from build123d import *

# Parameters (mm, degrees)
BASE_FLANGE1_DEPTH = 40
SKETCH2_R          = 1.5
SKETCH2_W          = 12.8
SKETCH2_H          = 3.5
SKETCH2_H_2        = 2
SKETCH2_H_3        = 4
SKETCH2_W_2        = 2
SKETCH2_H_4        = 9.5
CUT_EXTRUDE1_DEPTH = 33.4
CUT_EXTRUDE2_REACH = 68.173
SKETCH4_R          = 2


# Sheet-metal steps are written as plain solids
with BuildPart() as part:
    # Sketch1 → Base-Flange1 (new body)
    with BuildSketch(Plane(origin=(0, 0, 0), x_dir=(1, 0, 0), z_dir=(0, 1, 0))):
        with BuildLine():
            Line((14.7, 24), (14.7, -23.2634))
            ThreePointArc((14.7, -23.2634), (14.484254855, -23.784254855), (13.9634, -24))
            Line((13.9634, -24), (-13.9634, -24))
            ThreePointArc((-13.9634, -24), (-14.484254855, -23.784254855), (-14.7, -23.2634))
            Line((-14.7, -23.2634), (-14.7, 24))
            Line((-14.7, 24), (-16.7, 24))
            Line((-16.7, 24), (-16.7, -23.2634))
            ThreePointArc((-16.7, -23.2634), (-15.898468417, -25.198468417), (-13.9634, -26))
            Line((-13.9634, -26), (13.9634, -26))
            ThreePointArc((13.9634, -26), (15.898468417, -25.198468417), (16.7, -23.2634))
            Line((16.7, -23.2634), (16.7, 24))
            Line((16.7, 24), (14.7, 24))
        make_face()
    extrude(amount=BASE_FLANGE1_DEPTH)

    # Sketch2 → Cut-Extrude1 (cut)
    with BuildSketch(Plane.ZY.offset(16.7)):
        with Locations((-16.25, 12)):
            Circle(SKETCH2_R)
        with Locations((-16.25, 28)):
            Circle(SKETCH2_R)
        with Locations((21, 4)):
            Circle(SKETCH2_R)
        with Locations((21, 36)):
            Circle(SKETCH2_R)
        with Locations((-11, 4)):
            Circle(SKETCH2_R)
        with Locations((-11, 36)):
            Circle(SKETCH2_R)
        with Locations((10.15, 36)):
            Rectangle(SKETCH2_W, SKETCH2_H)
        with Locations((10.15, 17.5)):
            Rectangle(SKETCH2_W, SKETCH2_H_2)
        with Locations((10.15, 11)):
            Rectangle(SKETCH2_W, SKETCH2_H_3)
        with Locations((10.15, 29)):
            Rectangle(SKETCH2_W, SKETCH2_H_3)
        with Locations((10.15, 4)):
            Rectangle(SKETCH2_W, SKETCH2_H)
        with Locations((10.15, 22.5)):
            Rectangle(SKETCH2_W, SKETCH2_H_2)
        with Locations((-19.25, 8.75)):
            Rectangle(SKETCH2_W_2, SKETCH2_H_4)
        with Locations((-19.25, 31.25)):
            Rectangle(SKETCH2_W_2, SKETCH2_H_4)
    extrude(amount=-CUT_EXTRUDE1_DEPTH, mode=Mode.SUBTRACT)

    # Sketch4 → Cut-Extrude2 (cut, up to next)
    with BuildSketch(Plane.XY.offset(26), mode=Mode.PRIVATE) as cut_extrude2_sk1:
        with Locations((0, 10)):
            Circle(SKETCH4_R)
    cut_extrude2_tool1 = extrude(cut_extrude2_sk1.sketch, amount=-CUT_EXTRUDE2_REACH, mode=Mode.PRIVATE) & part.part
    # Sketch4 → Cut-Extrude2 (cut, up to next)
    with BuildSketch(Plane.XY.offset(26), mode=Mode.PRIVATE) as cut_extrude2_sk2:
        with Locations((0, 30)):
            Circle(SKETCH4_R)
    cut_extrude2_tool2 = extrude(cut_extrude2_sk2.sketch, amount=-CUT_EXTRUDE2_REACH, mode=Mode.PRIVATE) & part.part
    add(cut_extrude2_tool1.solids().sort_by_distance((0, 10, 26))[0], mode=Mode.SUBTRACT)
    add(cut_extrude2_tool2.solids().sort_by_distance((0, 30, 26))[0], mode=Mode.SUBTRACT)


solid = part.part
Verification items for the finished model (mm, model axes). A direction names the side the tool comes from. Round coordinates to 2 decimals unless told otherwise and drop trailing zeros. Loops run counter-clockwise (first coordinate to the right, second up) from the corner with the lowest first, then second, coordinate; pieces in that order, holes last. Notation, with made-up numbers: (88.5, 83.5) - (94.5, 83.5) arc R31 ccw to (94.5, 118.5) - close; hole circle Ø2 at (23.5, 75). An arc over 180 degrees is marked (long way). Answer in a Markdown table with one row per item. Add a question column.
Q1. Section check B-B on x = 0. Enter the section's corners in (y, z), plus the area to 3 significant figures.
Q2. Section check A-A on z = -11. Enter the section's corners in (x, y).
Q3. Tool access check on faces 1 (the face through (16, 20, -24)), 2 (the face through (-16, 31, 10)), 3 (the face through (14.7, 20, -1)). Record the directions out of +Z, -Z, +X, -X, +Y, -Y that give a thin tool (end or side, any length) a straight path to the whole face; none if there is none.
Q4. Section check C-C on z = 8.5. State how many separate pieces and enclosed holes the cut face has, plus the area to 3 significant figures.
Q5. Gauge pin test, flat ends, axial feed: pin 1 (1 mm diameter, centred on x = -1.5, y = 21, fed in from -Z); pin 2 (8 mm diameter, centred on x = -10.5, y = 27, fed in from -Z); pin 3 (1.6 mm diameter, centred on x = -15.5, y = 36.5, fed in from +Z). Record the tip position at first contact, or that the pin passes through.
Q6. Section check D-D on z = -16.5. Enter the section's corners in (x, y), plus the area to 3 significant figures.
Q7. Release check for a two-part mould opening along Z. For faces 4 (the face through (-15, 40, 5)), 5 (the face through (16, 27, 10)), 6 (the face through (-15.92, 19.72, 25.177)) record: pulls with the +Z half, pulls with the -Z half, needs draft (parallel to the pull), parting line crosses it, or undercut.
Q8. Material ranges on line 1 (Y direction, x = 15.4, z = -11); line 2 (X direction, y = 33, z = 10.5); line 3 (Y direction, x = 16, z = -16), recorded low to high.
Found:
| question | item | result |
|---|---|---|
| 1 | outline | (0, 24) - (8, 24) - (8, 26) - (0, 26) - close; (12, 24) - (28, 24) - (28, 26) - (12, 26) - close; (32, 24) - (40, 24) - (40, 26) - (32, 26) - close |
| 1 | area | 64.0 mm² |
| 2 | outline | (-16.7, 0) - (-14.7, 0) - (-14.7, 2.5) - (-16.7, 2.5) - close; (-16.7, 5.5) - (-14.7, 5.5) - (-14.7, 34.5) - (-16.7, 34.5) - close; (-16.7, 37.5) - (-14.7, 37.5) - (-14.7, 40) - (-16.7, 40) - close; (14.7, 0) - (16.7, 0) - (16.7, 2.5) - (14.7, 2.5) - close; (14.7, 5.5) - (16.7, 5.5) - (16.7, 34.5) - (14.7, 34.5) - close; (14.7, 37.5) - (16.7, 37.5) - (16.7, 40) - (14.7, 40) - close |
| 3 | face 1 | -Z, +X, -X, +Y, -Y |
| 3 | face 2 | +X, -X |
| 3 | face 3 | -Z, +Y, -Y |
| 4 | separate pieces | 14 |
| 4 | enclosed holes | 0 |
| 4 | area | 84.0 mm² |
| 5 | pin 1 | stops at z = 24 |
| 5 | pin 2 | stops at z = 23.77 |
| 5 | pin 3 | stops at z = 25.9 |
| 6 | outline | (-16.7, 0) - (-14.7, 0) - (-14.7, 10.52) - (-16.7, 10.52) - close; (-16.7, 13.48) - (-14.7, 13.48) - (-14.7, 26.52) - (-16.7, 26.52) - close; (-16.7, 29.48) - (-14.7, 29.48) - (-14.7, 40) - (-16.7, 40) - close; (14.7, 0) - (16.7, 0) - (16.7, 10.52) - (14.7, 10.52) - close; (14.7, 13.48) - (16.7, 13.48) - (16.7, 26.52) - (14.7, 26.52) - close; (14.7, 29.48) - (16.7, 29.48) - (16.7, 40) - (14.7, 40) - close |
| 6 | area | 136 mm² |
| 7 | face 4 | needs draft |
| 7 | face 5 | undercut |
| 7 | face 6 | pulls with the +Z half |
| 8 | line 1 | y = 0 to 2.5, 5.5 to 34.5, 37.5 to 40 |
| 8 | line 2 | x = -16.7 to -14.7, 14.7 to 16.7 |
| 8 | line 3 | y = 0 to 10.52, 13.48 to 26.52, 29.48 to 40 |
